Part model, mm, in its own coordinate system. Face numbers are marked on the shaded views. A direction names the side the tool comes from. Round coordinates to 2 decimals unless told otherwise and drop trailing zeros. Loops run counter-clockwise (first coordinate to the right, second up) from the corner with the lowest first, then second, coordinate; pieces in that order, holes last.
from build123d import *

# Parameters (mm, degrees)
SKETCH2_W               = 22.7
SKETCH2_H               = 23
BOSS_EXTRUDE1_DEPTH     = 12.2
BOSS_EXTRUDE2_START     = 17.106506393
BOSS_EXTRUDE2_OUTLINE_W = 12.2
BOSS_EXTRUDE2_OUTLINE_H = 4.9
BOSS_EXTRUDE2_DEPTH     = 2
SKETCH5_W               = 4.9
SKETCH5_H               = 2
BOSS_EXTRUDE4_DEPTH     = 12.2
SKETCH11_R              = 2.7
SKETCH11_R_2            = 0.95
BOSS_EXTRUDE6_DEPTH     = 27
SKETCH11_4_R            = 2.7
SKETCH11_4_R_2          = 0.95
BOSS_EXTRUDE7_DEPTH     = 30.3
CUT_EXTRUDE3_DEPTH      = 30.3
CUT_EXTRUDE4_DEPTH      = 30.3


# Read off the part's stored shape, not the designer's step: Boss-Extrude2
with BuildPart() as part:
    # Sketch2 → Boss-Extrude1 (new body)
    with BuildSketch(Plane(origin=(0, 0, 0), x_dir=(0, 0, -1), z_dir=(1, 0, 0))):
        with Locations((25.966711769, 11.60401504)):
            Rectangle(SKETCH2_W, SKETCH2_H)
    extrude(amount=BOSS_EXTRUDE1_DEPTH)

    # Boss-Extrude2 outline → Boss-Extrude2 (add)
    with BuildSketch(Plane(origin=(0, 0, 0), x_dir=(1, 0, 0), z_dir=(0, 1, 0)).offset(BOSS_EXTRUDE2_START)):
        with Locations((6.1, 12.166711769)):
            Rectangle(BOSS_EXTRUDE2_OUTLINE_W, BOSS_EXTRUDE2_OUTLINE_H)
    extrude(amount=BOSS_EXTRUDE2_DEPTH)

    # Sketch5 → Boss-Extrude4 (add)
    with BuildSketch(Plane(origin=(0, 0, 0), x_dir=(0, 0, -1), z_dir=(1, 0, 0))):
        with Locations((39.766711769, 18.10401504)):
            Rectangle(SKETCH5_W, SKETCH5_H)
    extrude(amount=BOSS_EXTRUDE4_DEPTH)

    # Sketch11 → Boss-Extrude6 (add)
    # profile 1 of 3: a face of its own
    with BuildSketch(Plane(origin=(0, 0, 0), x_dir=(1, 0, 0), z_dir=(0, 1, 0))):
        with BuildLine():
            ThreePointArc((8.818225568, 25.755828163), (6.081508494, 37.316683741), (3.414932422, 25.739448575))
            Line((3.414932422, 25.739448575), (3.414932422, 24.518358342))
            ThreePointArc((3.414932422, 24.518358342), (6.116578995, 21.816711769), (8.818225568, 24.518358342))
            Line((8.818225568, 24.518358342), (8.818225568, 25.755828163))
        make_face()
        with Locations((6.1, 31.216711769)):
            Circle(SKETCH11_R, mode=Mode.SUBTRACT)
    # profile 2 of 3: a face of its own
    with BuildSketch(Plane(origin=(0, 0, 0), x_dir=(1, 0, 0), z_dir=(0, 1, 0))):
        with Locations((6.1, 31.216711769)):
            Circle(SKETCH11_R)
        with Locations((6.1, 31.216711769)):
            Circle(SKETCH11_R_2, mode=Mode.SUBTRACT)
    # profile 3 of 3: a face of its own
    with BuildSketch(Plane(origin=(0, 0, 0), x_dir=(1, 0, 0), z_dir=(0, 1, 0))):
        with Locations((6.1, 31.216711769)):
            Circle(SKETCH11_R_2)
    extrude(amount=BOSS_EXTRUDE6_DEPTH)

    # Sketch11<4> → Boss-Extrude7 (add)
    with BuildSketch(Plane(origin=(0, 0, 0), x_dir=(1, 0, 0), z_dir=(0, 1, 0))):
        with Locations(Location((6.1, 31.216711769, 0), (0, 0, 90))):
            Circle(SKETCH11_4_R)
        with Locations(Location((6.1, 31.216711769, 0), (0, 0, 90))):
            Circle(SKETCH11_4_R_2, mode=Mode.SUBTRACT)
    extrude(amount=BOSS_EXTRUDE7_DEPTH)

    # Sketch13 → Cut-Extrude3 (cut)
    with BuildSketch(Plane(origin=(0, 0, 0), x_dir=(1, 0, 0), z_dir=(0, 1, 0))):
        with BuildLine():
            Line((5.528535179, 10.896085205), (5.528535179, 9.716711769))
            Line((5.528535179, 9.716711769), (6.671464821, 9.716711769))
            Line((6.671464821, 9.716711769), (6.671464821, 10.896085205))
            ThreePointArc((6.671464821, 10.896085205), (6.1, 12.716711769), (5.528535179, 10.896085205))
        make_face()
    extrude(amount=CUT_EXTRUDE3_DEPTH, mode=Mode.SUBTRACT)

    # Sketch16 → Cut-Extrude4 (cut)
    with BuildSketch(Plane(origin=(0, 0, 0), x_dir=(1, 0, 0), z_dir=(0, 1, 0))):
        with BuildLine():
            Line((5.646488236, 42.216711769), (6.553511764, 42.216711769))
            Line((6.553511764, 42.216711769), (6.553511764, 41.107962059))
            ThreePointArc((6.553511764, 41.107962059), (6.1, 39.216711769), (5.646488236, 41.107962059))
            Line((5.646488236, 41.107962059), (5.646488236, 42.216711769))
        make_face()
    extrude(amount=CUT_EXTRUDE4_DEPTH, mode=Mode.SUBTRACT)


solid = part.part
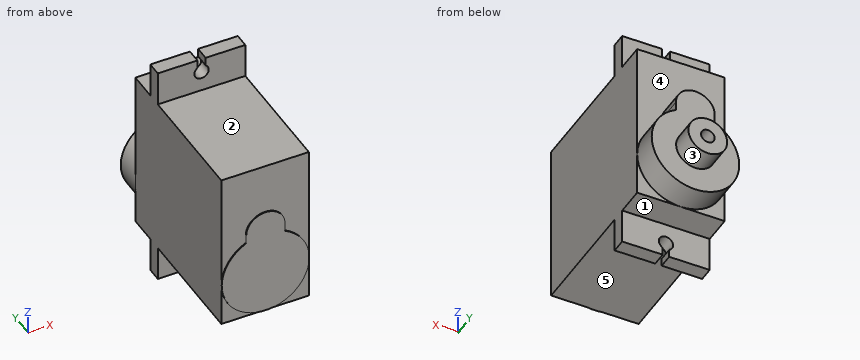
1) Wall check: line 1 along Z through (x, y) = (6.1, 18.4); line 2 along Y through (x, z) = (11, -21); line 3 along Y through (x, z) = (9.25, -36). Give the ranges that are in metal, low to high.
Values:
line 1: z = -39.22 to -12.72
line 2: y = 0.1 to 23.1
line 3: y = 0 to 27
2) Slice it at D-D, the plane z = -22.5. Give the cut face in (x, y).
Values:
outline: (0, 0.1) - (4.32, 0.1) - (4.32, 0) - (7.91, 0) - (7.91, 0.1) - (12.2, 0.1) - (12.2, 23.1) - (7.91, 23.1) - (7.91, 27) - (4.32, 27) - (4.32, 23.1) - (0, 23.1) - close
3) Slice it at A-A, the plane z = -36. Give the cut face in (x, y), then the cut area to 3 significant figures.
Values:
outline: (0, 0.1) - (2.31, 0.1) - (2.31, 0) - (9.89, 0) - (9.89, 0.1) - (12.2, 0.1) - (12.2, 23.1) - (9.89, 23.1) - (9.89, 27) - (2.31, 27) - (2.31, 23.1) - (0, 23.1) - close
area: 311 mm2
4) Slice it at C-C, the plane y = 7. Give the cut face in (x, z).
Values:
outline: (0, -37.32) - (12.2, -37.32) - (12.2, -14.62) - (0, -14.62) - close
5) Tool access for the marked faces 1, 2, 3, 4 and 5: list every direction of +Z, -Z, +X, -X, +Y, -Y with a clear straight run to the whole face (end or side of a thin tool).
Values:
face 1: -Z, +X, -X, +Y
face 2: +Z, +X, -X, -Y
face 3: +Y
face 4: +Z, +Y
face 5: -Z, +X, -X, -Y
6) Slice it at B-B, the plane x = 2. Give the cut face in (y, z), then the cut area to 3 significant figures.
Values:
outline: (0, -35.73) - (0.1, -35.73) - (0.1, -37.32) - (17.1, -37.32) - (17.1, -42.22) - (19.1, -42.22) - (19.1, -37.32) - (23.1, -37.32) - (23.1, -35.73) - (27, -35.73) - (27, -26.7) - (23.1, -26.7) - (23.1, -14.62) - (19.11, -14.62) - (19.11, -9.72) - (17.11, -9.72) - (17.11, -14.62) - (0.1, -14.62) - (0.1, -26.7) - (0, -26.7) - close
area: 578 mm2
7) Drop flat-ended pins along their axis: pin 1 Ø3 at (x, z) = (9, -35.5) entering from +Y; pin 2 Ø2.5 at (x, z) = (5, -12) entering from -Y; pin 3 Ø1.5 at (x, y) = (9.5, 23.5) entering from -Z. Give the stop position or say it passes through.
Values:
pin 1: stops at y = 27
pin 2: stops at y = 17.11
pin 3: stops at z = -37.32
